from build123d import *

# Parameters (mm, degrees)
SKETCH_1_W           = 27
SKETCH_1_H           = 40
EXTRUDE_1_DEPTH      = 10
SKETCH_2_W           = 25
SKETCH_2_H           = 31
CUT_EXTRUDE_1_DEPTH  = 9.2
CUT_EXTRUDE_2_DEPTH  = 9
SKETCH_8_W           = 25
SKETCH_8_H           = 2
SKETCH_8_H_2         = 1
CUT_EXTRUDE_7_DEPTH  = 3
SKETCH_9_W           = 8
SKETCH_9_H           = 2
CUT_EXTRUDE_8_DEPTH  = 6.2
CUT_EXTRUDE_9_DEPTH  = 0.65
SKETCH_10_3_W        = 1.2
SKETCH_10_3_H        = 1
CUT_EXTRUDE_10_DEPTH = 0.6
SKETCH_11_R          = 0.65
CUT_EXTRUDE_11_DEPTH = 6
SKETCH_12_R          = 0.6
CUT_EXTRUDE_12_DEPTH = 2
SKETCH_13_W          = 1
SKETCH_13_H          = 1
CUT_EXTRUDE_13_DEPTH = 0.6
FILLET_1_R           = 0.5
FILLET_2_R           = 0.5
FILLET_4_R           = 0.5
FILLET_5_R           = 0.5


with BuildPart() as part:
    # Sketch 1 → Extrude 1 (new body)
    with BuildSketch(Plane.XY):
        with Locations((13.5, 20)):
            Rectangle(SKETCH_1_W, SKETCH_1_H)
    extrude(amount=EXTRUDE_1_DEPTH)

    # Sketch 2 → Cut-Extrude 1 (cut)
    with BuildSketch(Plane.XY.offset(10)):
        with Locations((13.5, 17.5)):
            Rectangle(SKETCH_2_W, SKETCH_2_H)
    extrude(amount=-CUT_EXTRUDE_1_DEPTH, mode=Mode.SUBTRACT)

    # Sketch 3 → Cut-Extrude 2 (cut)
    with BuildSketch(Plane.XY.offset(10)):
        Polygon((1, 39), (9, 39), (9, 38), (11.5, 38), (11.5, 36), (9, 36), (1, 36), align=None)
        Polygon((15.5, 36), (15.5, 38), (18, 38), (18, 39), (26, 39), (26, 36), (18, 36), align=None)
    extrude(amount=-CUT_EXTRUDE_2_DEPTH, mode=Mode.SUBTRACT)

    # Sketch 8 → Cut-Extrude 7 (cut)
    with BuildSketch(Plane.XY.offset(10)):
        with Locations((13.5, 34)):
            Rectangle(SKETCH_8_W, SKETCH_8_H)
        with Locations((13.5, 1.5)):
            Rectangle(SKETCH_8_W, SKETCH_8_H_2)
    extrude(amount=-CUT_EXTRUDE_7_DEPTH, mode=Mode.SUBTRACT)

    # Sketch 9 → Cut-Extrude 8 (cut)
    with BuildSketch(Plane.XY.offset(7)):
        with Locations((5, 34)):
            Rectangle(SKETCH_9_W, SKETCH_9_H)
        with Locations((22, 34)):
            Rectangle(SKETCH_9_W, SKETCH_9_H)
    extrude(amount=-CUT_EXTRUDE_8_DEPTH, mode=Mode.SUBTRACT)

    # Sketch 10 → Cut-Extrude 9 (cut)
    with BuildSketch(Plane.XY.offset(10)):
        Polygon((14.15, 40), (13.5, 40), (12.85, 40), (12.85, 35), (13.5, 35), (14.15, 35), align=None)
    extrude(amount=-CUT_EXTRUDE_9_DEPTH, mode=Mode.SUBTRACT)

    # Sketch 10_3 → Cut-Extrude 10 (cut)
    with BuildSketch(Plane.XY.offset(10)):
        Polygon((12.9, 0), (13.5, 0), (14.1, 0), (14.1, 1), (13.5, 1), (12.9, 1), align=None)
        with Locations((2.1, 0.5)):
            Rectangle(SKETCH_10_3_W, SKETCH_10_3_H)
        with Locations((24.9, 0.5)):
            Rectangle(SKETCH_10_3_W, SKETCH_10_3_H)
    extrude(amount=-CUT_EXTRUDE_10_DEPTH, mode=Mode.SUBTRACT)

    # Sketch 11 → Cut-Extrude 11 (cut, through all)
    with BuildSketch(Plane.XZ.offset(-35)):
        with Locations((13.5, 9.35)):
            Circle(SKETCH_11_R)
    extrude(amount=-CUT_EXTRUDE_11_DEPTH, mode=Mode.SUBTRACT)

    # Sketch 12 → Cut-Extrude 12 (cut, through all)
    with BuildSketch(Plane(origin=(0, 1, 0), x_dir=(1, 0, 0), z_dir=(0, 1, 0))):
        with Locations((13.5, -9.4)):
            Circle(SKETCH_12_R)
        with Locations((24.9, -9.4)):
            Circle(SKETCH_12_R)
        with Locations((2.1, -9.4)):
            Circle(SKETCH_12_R)
    extrude(amount=-CUT_EXTRUDE_12_DEPTH, mode=Mode.SUBTRACT)

    # Sketch 13 → Cut-Extrude 13 (cut)
    with BuildSketch(Plane.XY.offset(10)):
        with Locations((11, 35.5)):
            Rectangle(SKETCH_13_W, SKETCH_13_H)
        with Locations((16, 35.5)):
            Rectangle(SKETCH_13_W, SKETCH_13_H)
    extrude(amount=-CUT_EXTRUDE_13_DEPTH, mode=Mode.SUBTRACT)

    # Fillet 1
    fillet_1_edges = [part.edges().sort_by_distance(p)[0] for p in [
        (18, 33, 3.9),
        (9, 33, 3.9),
    ]]
    fillet(fillet_1_edges, radius=FILLET_1_R)

    # Fillet 2
    fillet_2_edges = [part.edges().sort_by_distance(p)[0] for p in [
        (13.5, 40, 0),
        (27, 20, 0),
        (13.5, 0, 0),
        (0, 20, 0),
        (0, 40, 5),
        (27, 40, 5),
        (27, 0, 5),
        (0, 0, 5),
    ]]
    fillet(fillet_2_edges, radius=FILLET_2_R)

    # Fillet 4
    fillet_4_edges = [part.edges().sort_by_distance(p)[0] for p in [
        (9, 38, 5.5),
        (18, 38, 5.5),
    ]]
    fillet(fillet_4_edges, radius=FILLET_4_R)

    # Fillet 5
    fillet_5_edges = [part.edges().sort_by_distance(p)[0] for p in [
        (6.675, 40, 10),
        (19.2, 0, 10),
        (26, 0, 10),
        (7.8, 0, 10),
        (0, 20, 10),
        (20.325, 40, 10),
        (1, 0, 10),
        (0.146446609, 0.146446609, 10),
        (0.146446609, 39.853553391, 10),
        (27, 20, 10),
        (26.853553391, 0.146446609, 10),
        (26.853553391, 39.853553391, 10),
    ]]
    fillet(fillet_5_edges, radius=FILLET_5_R)


solid = part.part
Geometry: final body of the model. Coordinates: model frame, mm. A direction names the side the tool comes from. Give positions to 0.01 mm unless a question says otherwise; leave off trailing zeros. Loops run counter-clockwise (first coordinate to the right, second up) from the corner with the lowest first, then second, coordinate; pieces in that order, holes last. Notation, with made-up numbers: (-18, 73.5) -> (7, 73.5) arc R30 ccw to (7, 108.5) -> close; hole circle Ø9 at (-12.75, -34.75). An arc over 180 degrees is marked (long way). Put each result on its own line as item: value.
1. Cut plane A-A (z = 4). Count the separate pieces of the cut face and the enclosed holes in it, plus the area to 3 significant figures.
Taken from the geometry:
separate pieces: 1
enclosed holes: 3
area: 215 mm2
2. Ray query, line 1 along Y through (x, z) = (25.25, 8); line 2 along Y through (x, z) = (22.5, 5.25); line 3 along X through (y, z) = (38.5, 9.5). Return the intervals inside material, ascending. Write a range as [from, to].
Taken from the geometry:
line 1: y = [0, 1], [35, 36], [39, 40]
line 2: y = [0, 2], [35, 36], [39, 40]
line 3: x = [0, 1], [9, 12.85], [14.15, 18], [26, 27]
3. Cut plane D-D (z = 8.25). Return the cut outline in (x, y), plus the area to 3 significant figures.
Taken from the geometry:
outline: (0, 0.5) arc R0.5 ccw to (0.5, 0) -> (26.5, 0) arc R0.5 ccw to (27, 0.5) -> (27, 39.5) arc R0.5 ccw to (26.5, 40) -> (0.5, 40) arc R0.5 ccw to (0, 39.5) -> close; hole (1, 1) -> (26, 1) -> (26, 35) -> (1, 35) -> close; hole (1, 36) -> (11.5, 36) -> (11.5, 38) -> (9.5, 38) arc R0.5 cw to (9, 38.5) -> (9, 39) -> (1, 39) -> close; hole (15.5, 36) -> (26, 36) -> (26, 39) -> (18, 39) -> (18, 38.5) arc R0.5 cw to (17.5, 38) -> (15.5, 38) -> close
area: 172 mm2
4. Cut plane C-C (x = 2.1). Return the cut outline in (y, z).
Taken from the geometry:
outline: (0, 0.5) arc R0.5 ccw to (0.5, 0) -> (39.5, 0) arc R0.5 ccw to (40, 0.5) -> (40, 9.5) arc R0.5 ccw to (39.5, 10) -> (39, 10) -> (39, 1) -> (36, 1) -> (36, 10) -> (35, 10) -> (35, 0.8) -> (2, 0.8) -> (2, 7) -> (1, 7) -> (1, 8.8) -> (0, 8.8) -> close
5. Pull-direction query (Y, two-part tool) for faces 3 (the flat face through (0, 20, 5)), 4 (the flat face through (13, 40, 5)), 5 (the flat face through (13, 35, 8)); classes: released by +Y, released by -Y, zero draft, split by the parting line, or undercut.
Taken from the geometry:
face 3: zero draft
face 4: released by +Y
face 5: undercut
6. Set-up query: faces 1 (the flat face through (13, 20, 0)), 2 (the flat face through (13, 34, 7)). Return all of +Z, -Z, +X, -X, +Y, -Y with unobstructed straight access to the full face (end or side cutting, diameter ignored); none if empty.
Taken from the geometry:
face 1: -Z, +X, -X, +Y, -Y
face 2: +Z
7. Cut plane B-B (y = 30.5). Return the cut outline in (x, z), plus the area to 3 significant figures.
Taken from the geometry:
outline: (0, 0.5) arc R0.5 ccw to (0.5, 0) -> (26.5, 0) arc R0.5 ccw to (27, 0.5) -> (27, 9.5) arc R0.5 ccw to (26.5, 10) -> (26, 10) -> (26, 0.8) -> (1, 0.8) -> (1, 10) -> (0.5, 10) arc R0.5 ccw to (0, 9.5) -> close
area: 39.8 mm2
8. Pin query (flat end, axial travel): P1, Ø8, axis at x = 5.5, y = 14, coming from the +Z side; P2, Ø1.5, axis at x = 22.5, y = 38, coming from the +Z side. Return the tip coordinate at first contact, or that it passes through.
Taken from the geometry:
P1: stops at z = 0.8
P2: stops at z = 1
